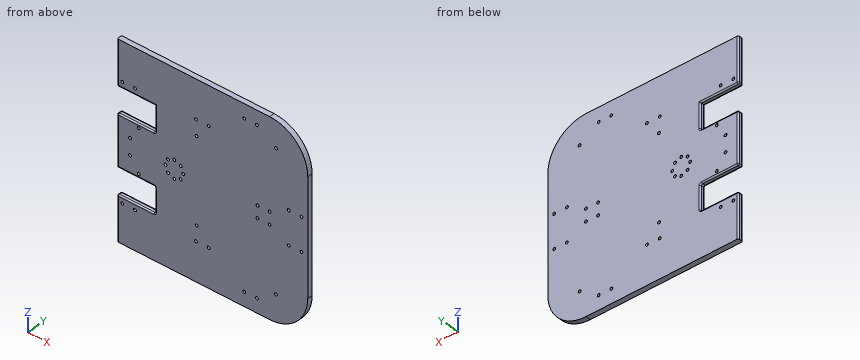
```python
from build123d import *

# Parameters (mm, degrees)
SKETCH_1_W                            = 300
SKETCH_1_H                            = 150
EXTRUDE_1_DEPTH                       = 4
FILLET_4_R                            = 30
FILLET_5_R                            = 30
FILLET_6_R                            = 30
FILLET_7_R                            = 30
HOLE_WIZARD_2_2_2_2_1_D               = 2.2
PATTERN_CIRCULAR_1_COUNT              = 8
MIRROR_1_COPY_1_D                     = 2.2
MIRROR_1_COPY_2_D                     = 2.2
MIRROR_1_COPY_3_D                     = 2.2
MIRROR_1_COPY_4_D                     = 2.2
MIRROR_1_COPY_5_D                     = 2.2
MIRROR_1_COPY_6_D                     = 2.2
MIRROR_1_COPY_7_D                     = 2.2
HOLE_WIZARD_2_2_2_2_2_D               = 2.2
HOLE_WIZARD_2_2_2_2_4_D               = 2.2
F_2_2_2_2_DIAMETER_HOLE1_D            = 2.2
MIRROR_5_AT_THE_SECOND_PLANE_COPY_1_D = 2.2
HOLE_WIZARD_2_2_2_2_6_D               = 2.2
F_2_2_2_2_DIAMETER_HOLE2_D            = 2.2
MIRROR_6_AT_THE_SECOND_PLANE_COPY_1_D = 2.2
F_2_2_2_2_DIAMETER_HOLE3_D            = 2.2
F_2_2_2_2_DIAMETER_HOLE4_D            = 2.2
MIRROR_8_AT_THE_SECOND_PLANE_COPY_1_D = 2.2
F_2_2_2_2_DIAMETER_HOLE5_D            = 2.2
MIRROR_9_AT_THE_SECOND_PLANE_COPY_1_D = 2.2
CUT_EXTRUDE_3_DEPTH                   = 168.752794314
CUT_EXTRUDE_3_DEPTH_BACK              = 168.752794314
SKETCH_25_W                           = 150
SKETCH_25_H                           = 4
SKETCH_28_W                           = 30
SKETCH_28_H                           = 20
CUT_EXTRUDE_4_DEPTH                   = 168.752794314
FILLET_8_R                            = 1


with BuildPart() as part:
    # 草图1 → 凸台-拉伸1 (new body)
    with BuildSketch(Plane(origin=(0, 0, 0), x_dir=(1, 0, 0), z_dir=(0, 1, 0))):
        Rectangle(SKETCH_1_W, SKETCH_1_H)
    extrude(amount=EXTRUDE_1_DEPTH)

    # 圆角4
    fillet_4_edges = [part.edges().sort_by_distance(p)[0] for p in [
        (-150, 2, 75),
    ]]
    fillet(fillet_4_edges, radius=FILLET_4_R)

    # 圆角5
    fillet_5_edges = [part.edges().sort_by_distance(p)[0] for p in [
        (-150, 2, -75),
    ]]
    fillet(fillet_5_edges, radius=FILLET_5_R)

    # 圆角6
    fillet_6_edges = [part.edges().sort_by_distance(p)[0] for p in [
        (150, 2, -75),
    ]]
    fillet(fillet_6_edges, radius=FILLET_6_R)

    # 圆角7
    fillet_7_edges = [part.edges().sort_by_distance(p)[0] for p in [
        (150, 2, 75),
    ]]
    fillet(fillet_7_edges, radius=FILLET_7_R)

    # Ø2.2 (2.2) 直径孔1 (through all)
    with Locations(Plane(origin=(0, 0, 0), x_dir=(-1, 0, 0), z_dir=(0, -1, 0))):
        with Locations((45, -7.02)):
            hole_wizard_2_2_2_2_1 = Hole(HOLE_WIZARD_2_2_2_2_1_D / 2)

    # 阵列(圆周)1: Ø2.2 (2.2) 直径孔1 ×8 about axis
    pattern_circular_1_axis = Axis((-45, 0, 0), (0, 1, 0))
    for i in range(1, PATTERN_CIRCULAR_1_COUNT):
        add(hole_wizard_2_2_2_2_1.rotate(pattern_circular_1_axis, i * 360 / PATTERN_CIRCULAR_1_COUNT), mode=Mode.SUBTRACT)

    # 镜向1: Ø2.2 (2.2) 直径孔1 across plane
    add(hole_wizard_2_2_2_2_1.mirror(Plane(origin=(0, 0, 0), x_dir=(0, 0, 1), z_dir=(1, 0, 0))), mode=Mode.SUBTRACT)

    # 镜向1 copy 1 (through all)
    with Locations(Plane(origin=(13.180194847, 0, -31.819805153), x_dir=(0.7071067811865476, 0, 0.7071067811865475), z_dir=(0, -1, 0))):
        with Locations((45, 7.02)):
            Hole(MIRROR_1_COPY_1_D / 2)

    # 镜向1 copy 2 (through all)
    with Locations(Plane(origin=(45, 0, -45), x_dir=(0, 0, 1), z_dir=(0, -1, 0))):
        with Locations((45, 7.02)):
            Hole(MIRROR_1_COPY_2_D / 2)

    # 镜向1 copy 3 (through all)
    with Locations(Plane(origin=(76.819805153, 0, -31.819805153), x_dir=(-0.7071067811865475, 0, 0.7071067811865476), z_dir=(0, -1, 0))):
        with Locations((45, 7.02)):
            Hole(MIRROR_1_COPY_3_D / 2)

    # 镜向1 copy 4 (through all)
    with Locations(Plane(origin=(90, 0, 0), x_dir=(-1, 0, 0), z_dir=(0, -1, 0))):
        with Locations((45, 7.02)):
            Hole(MIRROR_1_COPY_4_D / 2)

    # 镜向1 copy 5 (through all)
    with Locations(Plane(origin=(76.819805153, 0, 31.819805153), x_dir=(-0.7071067811865477, 0, -0.7071067811865475), z_dir=(0, -1, 0))):
        with Locations((45, 7.02)):
            Hole(MIRROR_1_COPY_5_D / 2)

    # 镜向1 copy 6 (through all)
    with Locations(Plane(origin=(45, 0, 45), x_dir=(0, 0, -1), z_dir=(0, -1, 0))):
        with Locations((45, 7.02)):
            Hole(MIRROR_1_COPY_6_D / 2)

    # 镜向1 copy 7 (through all)
    with Locations(Plane(origin=(13.180194847, 0, 31.819805153), x_dir=(0.7071067811865474, 0, -0.7071067811865477), z_dir=(0, -1, 0))):
        with Locations((45, 7.02)):
            Hole(MIRROR_1_COPY_7_D / 2)

    # Ø2.2 (2.2) 直径孔2 (through all)
    with Locations(Plane(origin=(0, 0, 0), x_dir=(-1, 0, 0), z_dir=(0, -1, 0))):
        with Locations((120, 4.78), (120, -4.775), (110.45, -4.775), (110.45, 4.78)):
            hole_wizard_2_2_2_2_2 = Hole(HOLE_WIZARD_2_2_2_2_2_D / 2)

    # 镜向2: Ø2.2 (2.2) 直径孔2 across plane
    add(hole_wizard_2_2_2_2_2.mirror(Plane(origin=(0, 0, 0), x_dir=(0, 0, 1), z_dir=(1, 0, 0))), mode=Mode.SUBTRACT)

    # Ø2.2 (2.2) 直径孔4 (through all)
    with Locations(Plane(origin=(0, 4, 0), x_dir=(1, 0, 0), z_dir=(0, 1, 0))):
        with Locations((100, -64), (110, -64), (-100, -64), (-110, -64)):
            hole_wizard_2_2_2_2_4 = Hole(HOLE_WIZARD_2_2_2_2_4_D / 2)

    # 镜向4: Ø2.2 (2.2) 直径孔4 across plane
    add(hole_wizard_2_2_2_2_4.mirror(Plane.XY), mode=Mode.SUBTRACT)

    # Ø2.2 (2.2) Diameter Hole1 (through all)
    with Locations(Plane(origin=(0, 4, 0), x_dir=(1, 0, 0), z_dir=(0, 1, 0))):
        with Locations((-125, 54)):
            f_2_2_2_2_diameter_hole1 = Hole(F_2_2_2_2_DIAMETER_HOLE1_D / 2)

    # 镜向5: Ø2.2 (2.2) Diameter Hole1 across plane
    add(f_2_2_2_2_diameter_hole1.mirror(Plane(origin=(0, 0, 0), x_dir=(0, 0, 1), z_dir=(1, 0, 0))), mode=Mode.SUBTRACT)

    # 镜向5 at the second plane: Ø2.2 (2.2) Diameter Hole1 across plane
    add(f_2_2_2_2_diameter_hole1.mirror(Plane.XY), mode=Mode.SUBTRACT)

    # 镜向5 at the second plane copy 1 (through all)
    with Locations(Plane(origin=(0, 4, 0), x_dir=(-1, 0, 0), z_dir=(0, 1, 0))):
        with Locations((-125, 54)):
            Hole(MIRROR_5_AT_THE_SECOND_PLANE_COPY_1_D / 2)

    # Ø2.2 (2.2) 直径孔6 (through all)
    with Locations(Plane(origin=(0, 4, 0), x_dir=(1, 0, 0), z_dir=(0, 1, 0))):
        with Locations((-62.5, 33), (-62.5, -33), (62.5, -33), (62.5, 33)):
            Hole(HOLE_WIZARD_2_2_2_2_6_D / 2)

    # Ø2.2 (2.2) Diameter Hole2 (through all)
    with Locations(Plane(origin=(0, 4, 0), x_dir=(1, 0, 0), z_dir=(0, 1, 0))):
        with Locations((-145, 13), (-135, 13)):
            f_2_2_2_2_diameter_hole2 = Hole(F_2_2_2_2_DIAMETER_HOLE2_D / 2)

    # 镜向6: Ø2.2 (2.2) Diameter Hole2 across plane
    add(f_2_2_2_2_diameter_hole2.mirror(Plane(origin=(0, 0, 0), x_dir=(0, 0, 1), z_dir=(1, 0, 0))), mode=Mode.SUBTRACT)

    # 镜向6 at the second plane: Ø2.2 (2.2) Diameter Hole2 across plane
    add(f_2_2_2_2_diameter_hole2.mirror(Plane.XY), mode=Mode.SUBTRACT)

    # 镜向6 at the second plane copy 1 (through all)
    with Locations(Plane(origin=(0, 4, 0), x_dir=(-1, 0, 0), z_dir=(0, 1, 0))):
        with Locations((-145, 13), (-135, 13)):
            Hole(MIRROR_6_AT_THE_SECOND_PLANE_COPY_1_D / 2)

    # Ø2.2 (2.2) Diameter Hole3 (through all)
    with Locations(Plane(origin=(0, 4, 0), x_dir=(1, 0, 0), z_dir=(0, 1, 0))):
        with Locations((-80, 45), (-70, 45), (-46, 45), (-36, 45), (4, 45), (14, 45), (62, 45), (72, 45)):
            f_2_2_2_2_diameter_hole3 = Hole(F_2_2_2_2_DIAMETER_HOLE3_D / 2)

    # 镜向7: Ø2.2 (2.2) Diameter Hole3 across plane
    add(f_2_2_2_2_diameter_hole3.mirror(Plane.XY), mode=Mode.SUBTRACT)

    # Ø2.2 (2.2) Diameter Hole4 (through all)
    with Locations(Plane.XZ):
        with Locations((-10.16, 6.35)):
            f_2_2_2_2_diameter_hole4 = Hole(F_2_2_2_2_DIAMETER_HOLE4_D / 2)

    # 镜向8: Ø2.2 (2.2) Diameter Hole4 across plane
    add(f_2_2_2_2_diameter_hole4.mirror(Plane.XY), mode=Mode.SUBTRACT)

    # 镜向8 at the second plane: Ø2.2 (2.2) Diameter Hole4 across plane
    add(f_2_2_2_2_diameter_hole4.mirror(Plane(origin=(0, 0, 0), x_dir=(0, 0, 1), z_dir=(1, 0, 0))), mode=Mode.SUBTRACT)

    # 镜向8 at the second plane copy 1 (through all)
    with Locations(Plane(origin=(0, 0, 0), x_dir=(-1, 0, 0), z_dir=(0, -1, 0))):
        with Locations((-10.16, 6.35)):
            Hole(MIRROR_8_AT_THE_SECOND_PLANE_COPY_1_D / 2)

    # Ø2.2 (2.2) Diameter Hole5 (through all)
    with Locations(Plane(origin=(0, 4, 0), x_dir=(1, 0, 0), z_dir=(0, 1, 0))):
        with Locations((-17, 17)):
            f_2_2_2_2_diameter_hole5 = Hole(F_2_2_2_2_DIAMETER_HOLE5_D / 2)

    # 镜向9: Ø2.2 (2.2) Diameter Hole5 across plane
    add(f_2_2_2_2_diameter_hole5.mirror(Plane.XY), mode=Mode.SUBTRACT)

    # 镜向9 at the second plane: Ø2.2 (2.2) Diameter Hole5 across plane
    add(f_2_2_2_2_diameter_hole5.mirror(Plane(origin=(0, 0, 0), x_dir=(0, 0, 1), z_dir=(1, 0, 0))), mode=Mode.SUBTRACT)

    # 镜向9 at the second plane copy 1 (through all)
    with Locations(Plane(origin=(0, 4, 0), x_dir=(-1, 0, 0), z_dir=(0, 1, 0))):
        with Locations((-17, 17)):
            Hole(MIRROR_9_AT_THE_SECOND_PLANE_COPY_1_D / 2)

    # 草图25 → 切除-拉伸3 (cut, two sides: drawn at the far end of the back side and taken through both)
    with BuildSketch(Plane.XY.offset(-CUT_EXTRUDE_3_DEPTH_BACK)):
        with Locations((-75, 2)):
            Rectangle(SKETCH_25_W, SKETCH_25_H)
    extrude(amount=CUT_EXTRUDE_3_DEPTH + CUT_EXTRUDE_3_DEPTH_BACK, mode=Mode.SUBTRACT)

    # 草图28 → 切除-拉伸4 (cut, through all)
    with BuildSketch(Plane(origin=(0, 4, 0), x_dir=(1, 0, 0), z_dir=(0, 1, 0))):
        with Locations((15, 30)):
            Rectangle(SKETCH_28_W, SKETCH_28_H)
    cut_extrude_4 = extrude(amount=-CUT_EXTRUDE_4_DEPTH, mode=Mode.SUBTRACT)

    # 镜向10: 切除-拉伸4 across plane
    add(cut_extrude_4.mirror(Plane.XY), mode=Mode.SUBTRACT)

    # 圆角8
    fillet_8_edges = [part.edges().sort_by_distance(p)[0] for p in [
        (0, 0, -57.5),
        (0, 4, -57.5),
        (0, 4, 0),
        (0, 0, 0),
        (30, 0, -30),
        (30, 2, -40),
        (15, 0, -20),
        (30, 2, -20),
        (0, 2, -20),
        (15, 0, -40),
        (0, 2, -40),
        (30, 4, -30),
        (15, 4, -40),
        (15, 4, -20),
        (0, 4, 57.5),
        (0, 0, 57.5),
        (30, 4, 30),
        (30, 2, 20),
        (15, 4, 40),
        (0, 2, 40),
        (15, 4, 20),
        (0, 2, 20),
        (30, 0, 30),
        (15, 0, 40),
        (15, 0, 20),
    ]]
    fillet(fillet_8_edges, radius=FILLET_8_R)


solid = part.part
```
Geometry: final body of the model. Coordinates: model frame, mm. Round coordinates to 2 decimals unless told otherwise and drop trailing zeros. Loops run counter-clockwise (first coordinate to the right, second up) from the corner with the lowest first, then second, coordinate; pieces in that order, holes last.
Item 1: Contact query for a flat-ended pin moving along its axis: P1, Ø1.5, axis at y = 1, z = 54, coming from the +X side. Output: stop coordinate, or through.
Checked values:
P1: stops at x = 148.84
Item 2: Section A-A, the plane z = -24. Output: boundary loops of the cut face in (x, y), plus the area to 3 significant figures.
Checked values:
outline: (30, 1) arc R1 ccw to (31, 0) - (150, 0) - (150, 4) - (31, 4) arc R1 ccw to (30, 3) - close
area: 480 mm2
Item 3: Line query: L1, parallel to Z at x = 28.5, y = 3; L2, parallel to Z at x = 45, y = 2.25; L3, parallel to Z at x = 17, y = 1.35. Output: solid intervals per line, ascending.
Checked values:
L1: z = -75 to -40, -20 to 20, 40 to 75
L2: z = -75 to -8.12, -5.92 to 5.92, 8.12 to 75
L3: z = -75 to -40, -20 to -18.1, -15.9 to 15.9, 18.1 to 20, 40 to 75
Item 4: Section B-B, the plane x = 141. Output: boundary loops of the cut face in (y, z).
Checked values:
outline: (0, -66.42) - (4, -66.42) - (4, 66.42) - (0, 66.42) - close
